Check sheet for the modelled part. Datum: model origin and axes. Units: mm. Face numbers are marked on the shaded views. A direction names the side the tool comes from. Give positions to 0.01 mm unless a question says otherwise; leave off trailing zeros. Write each loop counter-clockwise with the first axis right and the second up, starting at its lowest first coordinate (ties: lowest second). Pieces come first, ordered by that corner, then holes. Notation, with made-up numbers: M -3.75,-26 L 2.25,-26 A21 cw 2.25,-19 Z; hole C 60,-16.5 d7. An arc over 180 degrees is marked long. One line per item, written item: value. Start each with the question number.
from build123d import *

# Parameters (mm, degrees)
MODEL_R                 = 1.5
SALIENTE_EXTRUIR1_DEPTH = 3


with BuildPart() as part:
    # Model → Saliente-Extruir1 (new body)
    with BuildSketch(Plane.XY):
        with BuildLine():
            Line((198.613156537, 287.328333228), (193.181176022, 287.328333228))
            Line((193.181176022, 287.328333228), (184.260234476, 290.817294259))
            Line((184.260234476, 290.817294259), (169.975331899, 305.102196835))
            ThreePointArc((169.975331899, 305.102196835), (168.51542683, 306.077674216), (166.793351384, 306.42021632))
            Line((166.793351384, 306.42021632), (154.094067467, 306.461544477))
            Line((154.094067467, 306.461544477), (154.065429323, 306.461637676))
            ThreePointArc((154.065429323, 306.461637676), (152.38162222, 306.126707619), (150.954159485, 305.172907513))
            Line((150.954159485, 305.172907513), (150.812738129, 305.031486157))
            ThreePointArc((150.812738129, 305.031486157), (149.524007966, 301.92021632), (150.812738129, 298.808946483))
            Line((150.812738129, 298.808946483), (169.975331899, 279.646352713))
            ThreePointArc((169.975331899, 279.646352713), (171.435236969, 278.670875332), (173.157312415, 278.328333228))
            Line((173.157312415, 278.328333228), (198.613156537, 278.328333228))
            ThreePointArc((198.613156537, 278.328333228), (203.113156537, 282.828333228), (198.613156537, 287.328333228))
        make_face()
        with Locations((173.157312415, 282.828333228)):
            Circle(MODEL_R, mode=Mode.SUBTRACT)
        with Locations((166.793351384, 289.192294259)):
            Circle(MODEL_R, mode=Mode.SUBTRACT)
        with Locations((185.885234476, 282.828333228)):
            Circle(MODEL_R, mode=Mode.SUBTRACT)
        with Locations((198.613156537, 282.828333228)):
            Circle(MODEL_R, mode=Mode.SUBTRACT)
        with Locations((179.521273445, 289.192294259)):
            Circle(MODEL_R, mode=Mode.SUBTRACT)
        with Locations((160.429390353, 295.556255289)):
            Circle(MODEL_R, mode=Mode.SUBTRACT)
        with Locations((173.157312415, 295.556255289)):
            Circle(MODEL_R, mode=Mode.SUBTRACT)
        with Locations((154.065429323, 301.92021632)):
            Circle(MODEL_R, mode=Mode.SUBTRACT)
        with Locations((166.793351384, 301.92021632)):
            Circle(MODEL_R, mode=Mode.SUBTRACT)
    extrude(amount=SALIENTE_EXTRUIR1_DEPTH)


solid = part.part
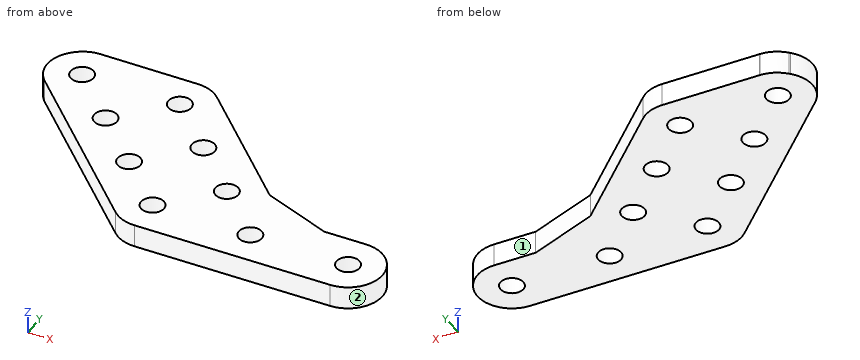
1) Tool access check on the marked faces 1 and 2. Record the directions out of +Z, -Z, +X, -X, +Y, -Y that give a thin tool (end or side, any length) a straight path to the whole face; none if there is none.
2) Cross-section at D-D (y = 285). Record the boundary of the cut face in (x, z), plus the area to 3 significant figures.
3) Cross-section at C-C (z = 0.7). State how many separate pieces and enclosed holes the cut face has, plus the area to 3 significant figures.
4) Cross-section at B-B (y = 290). Record the boundary of the cut face in (x, z).
5) Material ranges on L1, parallel to X at y = 300.75, z = 0.35; L2, parallel to X at y = 303.25, z = 2.15; L3, parallel to Y at x = 194, z = 0.5, recorded low to high. Write a range as from..to.
6) Cross-section at A-A (x = 160). Record the boundary of the cut face in (y, z), plus the area to 3 significant figures.
Data:
1. face 1: +Z, -Z, +X, +Y
1. face 2: +Z, -Z, +X
2. outline: M 164.62,0 L 202.55,0 L 202.55,3 L 164.62,3 Z
2. area: 114 mm2
3. separate pieces: 1
3. enclosed holes: 9
3. area: 725 mm2
4. outline: M 159.62,0 L 165.53,0 L 165.53,3 L 159.62,3 Z; M 168.06,0 L 178.26,0 L 178.26,3 L 168.06,3 Z; M 180.79,0 L 186.35,0 L 186.35,3 L 180.79,3 Z
5. L1: x = 149.68..153.13, 155..165.85, 167.73..174.33
5. L2: x = 149.73..153.37, 154.76..166.1, 167.49..171.83
5. L3: y = 278.33..287.33
6. outline: M 289.62,0 L 294.12,0 L 294.12,3 L 289.62,3 Z; M 296.99,0 L 306.44,0 L 306.44,3 L 296.99,3 Z
6. area: 41.8 mm2
